For this review, take the finished solid that the model builds, in its own axes (mm). Coordinates: 2 decimals unless noted, no trailing zeros. Loops run counter-clockwise (first coordinate to the right, second up) from the corner with the lowest first, then second, coordinate; pieces in that order, holes last. Notation, with made-up numbers: (-23, 1) -> (-9, 1) arc R11 ccw to (-9, 10) -> close; hole circle Ø1 at (72, 78). An arc over 180 degrees is marked (long way). Answer in a Markdown table with one row per item.
from build123d import *

# Parameters (mm, degrees)
F0_R     = 16.51
F0_W     = 152.420665353
F0_H     = 90.8812
F1_DEPTH = 3.175


# Not quite as in the source:
# - ends of sketch curves that miss each other by under 0.0002 mm in the source are joined
# - a feature names something its author has since deleted; it is built from what else it names


with BuildPart() as f1:
    # F0 (on Front) → F1 (new body)
    with BuildSketch(Plane.XZ):
        with BuildLine():
            Line((65.843271404, -64.4387074201), (72.172606051, -64.494198626))
            ThreePointArc((72.172606051, -64.494198626), (89.5045003647, -57.3150929397), (96.683606051, -39.983198626))
            Line((96.683606051, -39.983198626), (96.683606051, -30.0584486086))
            Line((96.683606051, -30.0584486086), (44.4719158113, 81.3992435336))
            Line((44.4719158113, 81.3992435336), (-29.9480052508, 81.3992435336))
            Line((-29.9480052508, 81.3992435336), (-35.9978974571, 50.6829957967))
            Line((-35.9978974571, 50.6829957967), (-19.4879078689, 50.6714224456))
            ThreePointArc((-19.4879078689, 50.6714224456), (-15.5812211009, 47.1637298884), (-13.9720730804, 42.1660573792))
            Line((-13.9720730804, 42.1660573792), (-5.4024819992, 38.3506346508))
            Line((-5.4024819992, 38.3506346508), (-2.9009456417, 36.1038269705))
            Line((-2.9009456417, 36.1038269705), (-2.3647786124, 27.9011076368))
            ThreePointArc((-2.3647786124, 27.9011076368), (3.4353485173, 23.5426794776), (4.3712937617, 16.3481414632))
            Line((4.3712937617, 16.3481414632), (4.2880776677, 1.0115236557))
            Line((4.2880776677, 1.0115236557), (-4.6405893252, -15.5276898319))
            Line((-4.6405893252, -15.5276898319), (-92.927393949, -15.5276898319))
            ThreePointArc((-92.927393949, -15.5276898319), (-117.3829027431, -39.983198626), (-92.927393949, -64.4387074201))
            Line((-92.927393949, -64.4387074201), (-86.577393949, -64.4387074201))
            Line((-86.577393949, -64.4387074201), (-86.577393949, -77.7312386201))
            Line((-86.577393949, -77.7312386201), (65.843271404, -77.7312386201))
            Line((65.843271404, -77.7312386201), (65.843271404, -64.4387074201))
        make_face()
        with Locations((11.6086210255, 54.3104703533)):
            Circle(F0_R, mode=Mode.SUBTRACT)
        with Locations((-10.3670612725, -123.1718386201)):
            Rectangle(F0_W, F0_H)
        with BuildLine():
            Line((65.843271404, -181.9049698201), (65.843271404, -168.6124386201))
            Line((65.843271404, -168.6124386201), (-86.577393949, -168.6124386201))
            Line((-86.577393949, -168.6124386201), (-86.577393949, -181.9049698201))
            Line((-86.577393949, -181.9049698201), (-92.927393949, -181.9049698201))
            ThreePointArc((-92.927393949, -181.9049698201), (-117.3829027431, -206.3604786142), (-92.927393949, -230.8159874083))
            Line((-92.927393949, -230.8159874083), (-4.6405893252, -230.8159874083))
            Line((-4.6405893252, -230.8159874083), (4.2880776677, -247.355200896))
            Line((4.2880776677, -247.355200896), (4.3712937617, -262.6918187035))
            ThreePointArc((4.3712937617, -262.6918187035), (3.4353485173, -269.8863567179), (-2.3647786124, -274.2447848771))
            Line((-2.3647786124, -274.2447848771), (-2.9009456417, -282.4475042108))
            Line((-2.9009456417, -282.4475042108), (-5.4024819992, -284.6943118911))
            Line((-5.4024819992, -284.6943118911), (-13.9720735102, -288.5097398532))
            ThreePointArc((-13.9720735102, -288.5097398532), (-15.5812211009, -293.5074071287), (-19.487905219, -297.0150996841))
            Line((-19.487905219, -297.0150996841), (-35.9978974571, -297.026673037))
            Line((-35.9978974571, -297.026673037), (-29.9480052508, -327.7429207739))
            Line((-29.9480052508, -327.7429207739), (44.4719158113, -327.7429207739))
            Line((44.4719158113, -327.7429207739), (96.683606051, -216.2852286317))
            Line((96.683606051, -216.2852286317), (96.683606051, -206.3604786142))
            ThreePointArc((96.683606051, -206.3604786142), (89.5045003647, -189.0285843006), (72.172606051, -181.8494786142))
            Line((72.172606051, -181.8494786142), (65.843271404, -181.9049698201))
        make_face()
        with Locations((11.6086210255, -300.6541475936)):
            Circle(F0_R, mode=Mode.SUBTRACT)
    extrude(amount=F1_DEPTH)


solid = f1.part
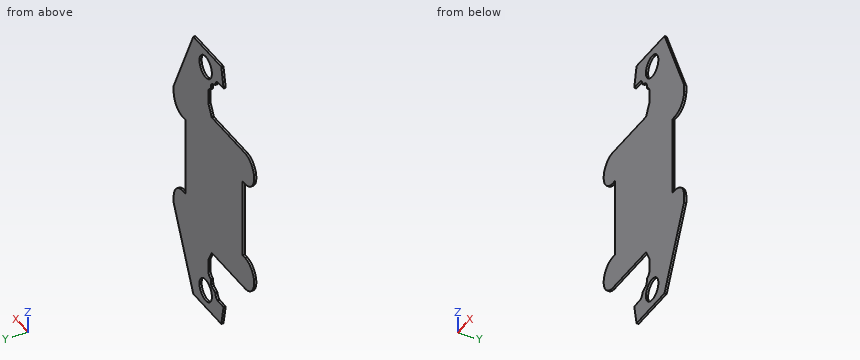
Item 1: Take a section at B-B, the plane y = -2.05. Count the separate pieces of the cut face and the enclosed holes in it, and give its area (3 significant figures).
Worked answers:
| item | result |
|---|---|
| separate pieces | 1 |
| enclosed holes | 2 |
| area | 51,500 mm² |
Item 2: Take a section at C-C, the plane z = -124. State the section outline as (x, y) points (3 decimals), and give its area (3 significant figures).
Worked answers:
| item | result |
|---|---|
| outline | (-86.577, -3.175) -> (65.843, -3.175) -> (65.843, 0) -> (-86.577, 0) -> close |
| area | 484 mm² |
Item 3: For L1, parallel to Z at x = 13, y = -0.3; L2, parallel to Z at x = 7.5, y = -1.6; L3, parallel to Z at x = -56, y = -0.85, list the stretches that pass through material, from the lowest coordinate up.
Worked answers:
| item | result |
|---|---|
| L1 | -327.74 to -317.11, -284.2 to 37.86, 70.76 to 81.4 |
| L2 | -327.74 to -316.64, -284.66 to 38.32, 70.3 to 81.4 |
| L3 | -230.82 to -15.53 |
Item 4: Take a section at A-A, the plane x = -102. State the section outline as (y, z) points (3 decimals), and give its area (3 significant figures).
Worked answers:
| item | result |
|---|---|
| outline | (-3.175, -229.071) -> (0, -229.071) -> (0, -183.65) -> (-3.175, -183.65) -> close; (-3.175, -62.694) -> (0, -62.694) -> (0, -17.273) -> (-3.175, -17.273) -> close |
| area | 288 mm² |
Item 5: Take a section at D-D, the plane x = 55. State the section outline as (y, z) points (3 decimals), and give its area (3 significant figures).
Worked answers:
| item | result |
|---|---|
| outline | (-3.175, -305.268) -> (0, -305.268) -> (0, 58.925) -> (-3.175, 58.925) -> close |
| area | 1,160 mm² |
Item 6: Insertion check: pin 1 (1 mm diameter, centred on x = -66.5, y = -2, fed in from +Z); pin 2 (1.6 mm diameter, centred on x = -58, y = -2, fed in from -Z). Each pin has a flat end and moves straight along its axis. Give the tip position at first contact, or say it passes through.
Worked answers:
| item | result |
|---|---|
| pin 1 | z = -15.53 |
| pin 2 | z = -230.82 |
